from build123d import *

# Parameters (mm, degrees)
SKETCH1_W                                       = 139.7
SKETCH1_H                                       = 152.4
BOSS_EXTRUDE1_DEPTH                             = 12
F_1_4_CLEARANCE_HOLE1_D                         = 6.7564
SKETCH8_W                                       = 139.7
SKETCH8_H                                       = 12
CUT_EXTRUDE2_DEPTH                              = 1.27
CBORE_FOR_10_SOCKET_HEAD_CAP_SCREW1_D           = 5.1054
CBORE_FOR_10_SOCKET_HEAD_CAP_SCREW1_CBORE_D     = 9.525
CBORE_FOR_10_SOCKET_HEAD_CAP_SCREW1_CBORE_DEPTH = 4.826


with BuildPart() as part:
    # Sketch1 → Boss-Extrude1 (new body)
    with BuildSketch(Plane(origin=(0, 0, 0), x_dir=(1, 0, 0), z_dir=(0, 1, 0))):
        Rectangle(SKETCH1_W, SKETCH1_H)
    extrude(amount=BOSS_EXTRUDE1_DEPTH)

    # 1/4 Clearance Hole1 (through all)
    with Locations(Plane(origin=(0, 12, 0), x_dir=(1, 0, 0), z_dir=(0, 1, 0))):
        with Locations((-50.8, 50.8), (50.8, 50.8), (50.8, -50.8), (-50.8, -50.8)):
            Hole(F_1_4_CLEARANCE_HOLE1_D / 2)

    # Sketch8 → Cut-Extrude2 (cut)
    with BuildSketch(Plane(origin=(0, 12, 0), x_dir=(1, 0, 0), z_dir=(0, 1, 0))):
        with Locations((0, 35.275)):
            Rectangle(SKETCH8_W, SKETCH8_H)
        with Locations((0, -16.225)):
            Rectangle(SKETCH8_W, SKETCH8_H)
    extrude(amount=-CUT_EXTRUDE2_DEPTH, mode=Mode.SUBTRACT)

    # CBORE for #10 Socket Head Cap Screw1 (through all)
    with Locations(Plane(origin=(0, 0, 0), x_dir=(-1, 0, 0), z_dir=(0, -1, 0))):
        with Locations((-50.8, 35.275), (0, 35.275), (50.8, 35.275), (50.8, -16.225), (0, -16.225), (-50.8, -16.225)):
            CounterBoreHole(CBORE_FOR_10_SOCKET_HEAD_CAP_SCREW1_D / 2, CBORE_FOR_10_SOCKET_HEAD_CAP_SCREW1_CBORE_D / 2, CBORE_FOR_10_SOCKET_HEAD_CAP_SCREW1_CBORE_DEPTH)


solid = part.part
Geometry: final body of the model. Coordinates: model frame, mm. A direction names the side the tool comes from. Coordinates: 2 decimals unless noted, no trailing zeros. Order: outer loops, then holes, each group sorted by start corner. A loop starts at its lowest first (then second) coordinate and runs counter-clockwise, first axis right, second up. Notation, with made-up numbers: M 50,81.5 L 108,81.5 A14 ccw 108,85.5 Z; hole C 78,44.5 d10. An arc over 180 degrees is marked long. One line per question, with ' | ' between items. Start each with the question number.
Item 1: Ray query, probe 1 along Z at (x, y) = (0, 3); probe 2 along Z at (x, y) = (0, 6.85); probe 3 along Z at (x, y) = (-50.8, 4.75). Return the intervals inside material, ascending. Write a range as [from, to].
Item 2: Pin query (flat end, axial travel): pin 1 Ø4 at (x, z) = (50.8, 50.8) entering from -Y; pin 2 Ø6.5 at (x, z) = (-50.8, -35.275) entering from +Y; pin 3 Ø6 at (x, z) = (0, 16.225) entering from -Y. Return the tip coordinate at first contact, or that it passes through.
Item 3: Cut plane C-C, the plane x = 37. Return the cut outline in (y, z) (3 decimals), then the cut area to 3 significant figures.
Item 4: Set-up query: faces 1 (the flat face through (-1, 10.73, -38)), 2 (the flat face through (-1, 12, -10)), 3 (the flat face through (48.8, 4.826, 18.3)). Return all of +Z, -Z, +X, -X, +Y, -Y with unobstructed straight access to the full face (end or side cutting, diameter ignored); none if empty.
Item 5: Cut plane A-A, the plane x = 0. Return the cut outline in (y, z) (1 decimal).
Item 6: Cut plane B-B, the plane z = 50.8. Return the cut outline in (x, y), then the cut area to 3 significant figures.
Item 7: Draft query along Z for faces 4 (the flat face through (-1, 10.73, 13)), 5 (the cylindrical face through (-50.07, 5.92, 54.1)), 6 (the flat face through (-1, 6, 76.2)), 7 (the flat face through (69.85, 6, 1)). Return one class per face: released by +Z, released by -Z, zero draft, split by the parting line, or undercut.
A:
1) probe 1: z = [-76.2, -40.04], [-30.51, 11.46], [20.99, 76.2] | probe 2: z = [-76.2, -37.83], [-32.72, 13.67], [18.78, 76.2] | probe 3: z = [-76.2, -54.18], [-47.42, -40.04], [-30.51, 11.46], [20.99, 47.42], [54.18, 76.2]
2) pin 1: passes through | pin 2: stops at y = 10.73 | pin 3: stops at y = 4.83
3) outline: M 0,-76.2 L 12,-76.2 L 12,-41.275 L 10.73,-41.275 L 10.73,-29.275 L 12,-29.275 L 12,10.225 L 10.73,10.225 L 10.73,22.225 L 12,22.225 L 12,76.2 L 0,76.2 Z | area: 1,800 mm2
4) face 1: +X, -X, +Y | face 2: +Z, -Z, +X, -X, +Y | face 3: -Y
5) outline: M 0,-76.2 L 12,-76.2 L 12,-41.3 L 10.7,-41.3 L 10.7,-37.8 L 4.8,-37.8 L 4.8,-40 L 0,-40 Z; M 0,-30.5 L 4.8,-30.5 L 4.8,-32.7 L 10.7,-32.7 L 10.7,-29.3 L 12,-29.3 L 12,10.2 L 10.7,10.2 L 10.7,13.7 L 4.8,13.7 L 4.8,11.5 L 0,11.5 Z; M 0,21 L 4.8,21 L 4.8,18.8 L 10.7,18.8 L 10.7,22.2 L 12,22.2 L 12,76.2 L 0,76.2 Z
6) outline: M -69.85,0 L -54.18,0 L -54.18,12 L -69.85,12 Z; M -47.42,0 L 47.42,0 L 47.42,12 L -47.42,12 Z; M 54.18,0 L 69.85,0 L 69.85,12 L 54.18,12 Z | area: 1,510 mm2
7) face 4: undercut | face 5: undercut | face 6: released by +Z | face 7: zero draft
